The listing builds one solid part. Answer for the finished solid, in the listing's coordinates (mm). A direction names the side the tool comes from. Coordinates: 2 decimals unless noted, no trailing zeros. Order: outer loops, then holes, each group sorted by start corner. A loop starts at its lowest first (then second) coordinate and runs counter-clockwise, first axis right, second up. Notation, with made-up numbers: (-33, -18.5) -> (-16, -18.5) arc R24 ccw to (-16, 8.5) -> close; hole circle Ø8 at (74, -37.75). An arc over 180 degrees is marked (long way). Answer in a Markdown table with one row per item.
```python
from build123d import *

# Parameters (mm, degrees)
SKETCH_1_W          = 15
SKETCH_1_H          = 10
SKETCH_1_W_2        = 12.6
SKETCH_1_H_2        = 7.6
EXTRUDE_1_DEPTH     = 110
SKETCH_2_R          = 1.6
CUT_EXTRUDE_1_DEPTH = 100
SKETCH_3_R          = 1.6
CUT_EXTRUDE_2_DEPTH = 15
SKETCH_5_W          = 15
SKETCH_5_H          = 10
CUT_EXTRUDE_4_DEPTH = 14.5
SKETCH_6_R          = 1.6
CUT_EXTRUDE_5_DEPTH = 15
CUT_EXTRUDE_6_DEPTH = 15


with BuildPart() as part:
    # ｽｹｯﾁ1 → ﾎﾞｽ - 押し出し1 (new, symmetric)
    with BuildSketch(Plane(origin=(0, 0, 0), x_dir=(1, 0, 0), z_dir=(0, 1, 0))):
        Rectangle(SKETCH_1_W, SKETCH_1_H)
        Rectangle(SKETCH_1_W_2, SKETCH_1_H_2, mode=Mode.SUBTRACT)
    extrude(amount=EXTRUDE_1_DEPTH, both=True)

    # ｽｹｯﾁ2 → ｶｯﾄ - 押し出し1 (cut)
    with BuildSketch(Plane(origin=(0, 0, -5), x_dir=(-1, 0, 0), z_dir=(0, 0, -1))):
        with Locations((0, -85)):
            Circle(SKETCH_2_R)
        with Locations((0, -105)):
            Circle(SKETCH_2_R)
    extrude(amount=-CUT_EXTRUDE_1_DEPTH, mode=Mode.SUBTRACT)

    # ｽｹｯﾁ3 → ｶｯﾄ - 押し出し2 (cut)
    with BuildSketch(Plane.ZY.offset(7.5)):
        with Locations((-0.2, -74)):
            Circle(SKETCH_3_R)
        with Locations((-0.2, -34)):
            Circle(SKETCH_3_R)
    extrude(amount=-CUT_EXTRUDE_2_DEPTH, mode=Mode.SUBTRACT)

    # ｽｹｯﾁ5 → ｶｯﾄ - 押し出し4 (cut)
    with BuildSketch(Plane(origin=(0, 110, 0), x_dir=(1, 0, 0), z_dir=(0, 1, 0))):
        Rectangle(SKETCH_5_W, SKETCH_5_H)
    extrude(amount=-CUT_EXTRUDE_4_DEPTH, mode=Mode.SUBTRACT)

    # ｽｹｯﾁ6 → ｶｯﾄ - 押し出し5 (cut)
    with BuildSketch(Plane(origin=(0, 0, -5), x_dir=(-1, 0, 0), z_dir=(0, 0, -1))):
        with Locations((0, 56.66)):
            Circle(SKETCH_6_R)
        with Locations((0, 76.66)):
            Circle(SKETCH_6_R)
    extrude(amount=-CUT_EXTRUDE_5_DEPTH, mode=Mode.SUBTRACT)

    # ｽｹｯﾁ7 → ｶｯﾄ - 押し出し6 (cut)
    with BuildSketch(Plane.ZY.offset(7.5)):
        with BuildLine():
            ThreePointArc((0, 93.15), (-1.65, 91.5), (0, 89.85))
            ThreePointArc((0, 89.85), (1.65, 91.5), (0, 93.15))
        make_face()
    extrude(amount=-CUT_EXTRUDE_6_DEPTH, mode=Mode.SUBTRACT)


solid = part.part
```
(1) A cutting plane is placed at B-B, the plane y = 39. Determine the outline of the cut face in (x, z), then the cut area to 3 significant figures.
Check values:
| item | result |
|---|---|
| outline | (-7.5, -5) -> (7.5, -5) -> (7.5, 5) -> (-7.5, 5) -> close; hole (-6.3, -3.8) -> (6.3, -3.8) -> (6.3, 3.8) -> (-6.3, 3.8) -> close |
| area | 54.2 mm² |
(2) For a pull along X with two mould halves and no side action, classify faces 1 (the flat face through (7.5, -6, 0)), 2 (the flat face through (-7.5, -6, 0)), 3 (the cylindrical face through (0.208, 78.246, 4.392)), 4 (the cylindrical face through (-6.91, -35.42, 0.54)) as released by +X, released by -X, zero draft, split by the parting line, or undercut.
Check values:
| item | result |
|---|---|
| face 1 | released by +X |
| face 2 | released by -X |
| face 3 | undercut |
| face 4 | zero draft |
(3) Find the intervals of material crossed by line 1 along Y through (x, z) = (-7, 0); line 2 along X through (y, z) = (-19, -2); line 3 along Z through (x, y) = (2, 3.5), in increasing order. Write a range as from..to.
Check values:
| item | result |
|---|---|
| line 1 | -110..-75.59, -72.41..-35.59, -32.41..89.85, 93.15..95.5 |
| line 2 | -7.5..-6.3, 6.3..7.5 |
| line 3 | -5..-3.8, 3.8..5 |
(4) Flat-ended cylindrical pins translate along their axes: pin 1 (5 mm diameter, centred on x = 0, y = 76.66, fed in from +Z); pin 2 (3 mm diameter, centred on x = 0, y = -105, fed in from -Z). Find the tip coordinate at first contact, or state that the pin passes through.
Check values:
| item | result |
|---|---|
| pin 1 | z = 5 |
| pin 2 | through |
(5) Which of the six approach directions +Z, -Z, +X, -X, +Y, -Y give full straight-line access (tool end or side, diameter ignored) to faces 5 (the flat face through (0, 95.5, 4)), 6 (the flat face through (0, -6, -3.8))?
Check values:
| item | result |
|---|---|
| face 5 | +Z, -Z, +X, -X, +Y |
| face 6 | +Y, -Y |
(6) A cutting plane is placed at A-A, the plane x = 3.75. Determine the outline of the cut face in (y, z), then the cut area to 3 significant figures.
Check values:
| item | result |
|---|---|
| outline | (-110, -5) -> (95.5, -5) -> (95.5, -3.8) -> (-110, -3.8) -> close; (-110, 3.8) -> (95.5, 3.8) -> (95.5, 5) -> (-110, 5) -> close |
| area | 493 mm² |
